For this review, take the finished solid that the model builds, in its own axes (mm). Face numbers are marked on the shaded views. Give positions to 0.01 mm unless a question says otherwise; leave off trailing zeros. Write each loop counter-clockwise with the first axis right and the second up, starting at its lowest first coordinate (ties: lowest second). Pieces come first, ordered by that corner, then holes.
Q1. Mouldability with a two-part tool opening along Y and no side actions: class the marked faces 1, 2 and 3 as released by +Y, released by -Y, zero draft, split by the parting line, or undercut.
Q2. We need section A-A (y = 4). Write out the cut boundary in (x, z), then the cut area to 3 significant figures.
Q3. We need section C-C (x = 20.5). Write out the cut boundary in (y, z).
Q4. We need section D-D (x = 16.75). Write out the cut boundary in (y, z), then the cut area to 3 significant figures.
Q5. Insertion check: P1, Ø1.8, axis at y = 4, z = 4, coming from the -X side. The pin has a flat end and moves straight along its axis. Give the tip position at first contact, or say it passes through.
Q6. For line 1 (X direction, y = 2.75, z = 4); line 2 (Y direction, x = 4.5, z = 4); line 3 (Y direction, x = 2, z = 4.5), list the stretches that pass through material, from the lowest coordinate up.
Q7. We need section B-B (z = 4). Write out the cut boundary in (x, y), then the cut area to 3 significant figures.
```python
from build123d import *

# Parameters (mm, degrees)
CROQUIS1_W              = 29
CROQUIS1_H              = 8
SALIENTE_EXTRUIR1_DEPTH = 8
CROQUIS4_R              = 1.75
CORTAR_EXTRUIR1_DEPTH   = 9
REDONDEO1_R             = 2
CROQUIS5_R              = 1.5
CORTAR_EXTRUIR2_DEPTH   = 9.5
CROQUIS6_R              = 1.5
CORTAR_EXTRUIR3_DEPTH   = 9.5


with BuildPart() as part:
    # Croquis1 → Saliente-Extruir1 (new body)
    with BuildSketch(Plane.XY):
        with Locations((14.5, 4)):
            Rectangle(CROQUIS1_W, CROQUIS1_H)
    extrude(amount=SALIENTE_EXTRUIR1_DEPTH)

    # Croquis4 → Cortar-Extruir1 (cut, through all)
    with BuildSketch(Plane(origin=(0, 8, 0), x_dir=(1, 0, 0), z_dir=(0, 1, 0))):
        with Locations((14.5, -4)):
            Circle(CROQUIS4_R)
    extrude(amount=-CORTAR_EXTRUIR1_DEPTH, mode=Mode.SUBTRACT)

    # Redondeo1
    redondeo1_edges = [part.edges().sort_by_distance(p)[0] for p in [
        (29, 4, 8),
        (14.5, 8, 8),
        (0, 4, 8),
        (14.5, 8, 0),
        (29, 4, 0),
        (14.5, 0, 0),
        (0, 4, 0),
        (0, 8, 4),
        (29, 8, 4),
        (29, 0, 4),
        (0, 0, 4),
        (14.5, 0, 8),
    ]]
    fillet(redondeo1_edges, radius=REDONDEO1_R)

    # Croquis5 → Cortar-Extruir2 (cut)
    with BuildSketch(Plane(origin=(29, 0, 0), x_dir=(0, 0, -1), z_dir=(1, 0, 0))):
        with Locations((-4, 4)):
            Circle(CROQUIS5_R)
    extrude(amount=-CORTAR_EXTRUIR2_DEPTH, mode=Mode.SUBTRACT)

    # Croquis6 → Cortar-Extruir3 (cut)
    with BuildSketch(Plane.ZY):
        with Locations((4, 4)):
            Circle(CROQUIS6_R)
    extrude(amount=-CORTAR_EXTRUIR3_DEPTH, mode=Mode.SUBTRACT)


solid = part.part
```
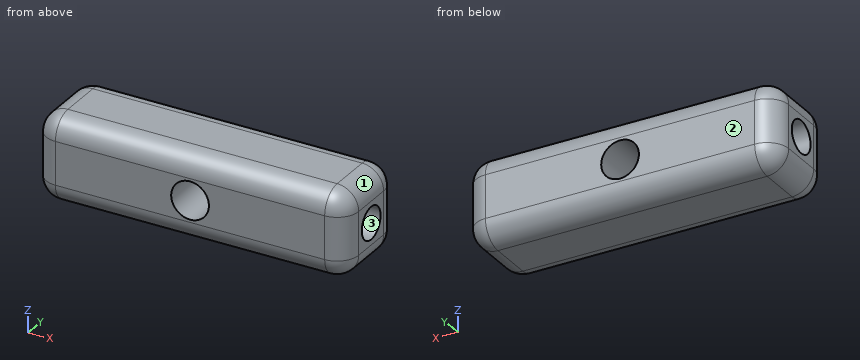
Computed:
1. face 1: zero draft
1. face 2: released by +Y
1. face 3: undercut
2. outline: (0, 2) arc R2 ccw to (2, 0) - (27, 0) arc R2 ccw to (29, 2) - (29, 2.5) - (19.5, 2.5) - (19.5, 5.5) - (29, 5.5) - (29, 6) arc R2 ccw to (27, 8) - (2, 8) arc R2 ccw to (0, 6) - (0, 5.5) - (9.5, 5.5) - (9.5, 2.5) - (0, 2.5) - close; hole circle Ø3.5 at (14.5, 4)
2. area: 162 mm2
3. outline: (0, 2) arc R2 ccw to (2, 0) - (6, 0) arc R2 ccw to (8, 2) - (8, 6) arc R2 ccw to (6, 8) - (2, 8) arc R2 ccw to (0, 6) - close; hole circle Ø3 at (4, 4)
4. outline: (0, 2) arc R2 ccw to (2, 0) - (6, 0) arc R2 ccw to (8, 2) - (8, 6) arc R2 ccw to (6, 8) - (2, 8) arc R2 ccw to (0, 6) - close
4. area: 60.6 mm2
5. P1: stops at x = 9.5
6. line 1: x = 9.5 to 12.75, 16.25 to 19.5
6. line 2: y = 0 to 2.5, 5.5 to 8
6. line 3: y = 0 to 2.59, 5.41 to 8
7. outline: (0, 2) arc R2 ccw to (2, 0) - (12.75, 0) - (12.75, 8) - (2, 8) arc R2 ccw to (0, 6) - (0, 5.5) - (9.5, 5.5) - (9.5, 2.5) - (0, 2.5) - close; (16.25, 0) - (27, 0) arc R2 ccw to (29, 2) - (29, 2.5) - (19.5, 2.5) - (19.5, 5.5) - (29, 5.5) - (29, 6) arc R2 ccw to (27, 8) - (16.25, 8) - close
7. area: 144 mm2
